Read the model definition and answer for the solid it produces. Units are mm, in the model's axes. Round coordinates to 2 decimals unless told otherwise and drop trailing zeros. Write each loop counter-clockwise with the first axis right and the second up, starting at its lowest first coordinate (ties: lowest second). Pieces come first, ordered by that corner, then holes. Notation, with made-up numbers: M 40,-24.75 L 55,-24.75 A19 cw 55,-5.75 Z; hole C 42,59.5 d6. An arc over 180 degrees is marked long. Use one line per item in the form item = value. Start each with the question number.
```python
from build123d import *

# Parameters (mm, degrees)
F0_W          = 15
F0_H          = 1
F2_R          = 0.5
F3_DEPTH      = 31.001
F3_DEPTH_BACK = 31.001
F4_R          = 0.5
F5_DEPTH      = 31.0010001
F5_DEPTH_BACK = 31.0010001


with BuildPart() as f1:
    # F0 (on Right) → F1 (revolve)
    with BuildSketch(Plane.YZ):
        with Locations((-1.5, 30.5)):
            Rectangle(F0_W, F0_H)
    revolve(axis=Axis((0, 3, 0), (0, -1, 0)))

    # F2 (on Right) → F3 (cut, two sides)
    with BuildSketch(Plane.YZ) as f3_sk:
        Circle(F2_R)
    extrude(amount=-F3_DEPTH, mode=Mode.SUBTRACT)
    extrude(f3_sk.sketch, amount=F3_DEPTH_BACK, mode=Mode.SUBTRACT)

    # F4 (on Top) → F5 (cut, two sides)
    with BuildSketch(Plane.XY) as f5_sk:
        with Locations((0, -5)):
            Circle(F4_R)
    extrude(amount=-F5_DEPTH, mode=Mode.SUBTRACT)
    extrude(f5_sk.sketch, amount=F5_DEPTH_BACK, mode=Mode.SUBTRACT)


solid = f1.part
```
Q1. Each of these flat-tipped pins is pushed along its axis until it touches: pin 1 Ø6 at (y, z) = (-1.5, 17) entering from +X; pin 2 Ø2 at (y, z) = (1.5, -19.5) entering from +X. Where does it stop, or does it pass through?
Q2. Find section C-C on y = 2.5. Write down the section's boundary in (x, z).
Q3. Straight lines are drawn through the part: line 1 (Z direction, x = 0, y = 2.25); line 2 (X direction, y = -8.25, z = -24). For each, find the intervals that lie inside material, in ascending order. Write a range as [from, to].
Q4. For a pull along X with two mould halves and no side action, classify faces 1 (the face through (-30.736, -1.395, -4.036)), 2 (the face through (-28, 6, 12)), 3 (the face through (-1.32, -1.39, -29.97)) as +X half, -X half, draft (parallel to the pull), parting line (faces both ways), or undercut.
Q5. Find section A-A on z = 9. Write down the section's boundary in (x, y), and give its area (3 significant figures).
Q6. Find section B-B on x = -5. Write down the section's boundary in (y, z).
Response:
q1.pin_1 = 27.66
q1.pin_2 = 24.87
q2.outline = C 0,0 d62; hole C 0,0 d60
q3.line_1 = [-31, -30], [30, 31]
q3.line_2 = [-19.62, -18], [18, 19.62]
q4.face_1 = parting line
q4.face_2 = draft
q4.face_3 = undercut
q5.outline = M -29.66,-9 L -28.62,-9 L -28.62,6 L -29.66,6 Z; M 28.62,-9 L 29.66,-9 L 29.66,6 L 28.62,6 Z
q5.area = 31.4 mm²
q6.outline = M -9,-30.59 L 6,-30.59 L 6,-29.58 L -9,-29.58 Z; M -9,29.58 L 6,29.58 L 6,30.59 L -9,30.59 Z
